Verification items for the finished model (mm, model axes). Face numbers are marked on the shaded views. A direction names the side the tool comes from. Coordinates: 2 decimals unless noted, no trailing zeros. Write each loop counter-clockwise with the first axis right and the second up, starting at its lowest first coordinate (ties: lowest second). Pieces come first, ordered by that corner, then holes. Notation, with made-up numbers: (47, -23.5) -> (100, -23.5) arc R11 cw to (100, -9.5) -> close; hole circle Ø3 at (-38, 61). An arc over 180 degrees is marked (long way). Answer in a Markdown table with one row per item.
```python
from build123d import *

# Parameters (mm, degrees)
BOSS_EXTRUDE1_DEPTH     = 82.55
SKETCH4_W               = 139.7
SKETCH4_H               = 139.7
SKETCH4_W_2             = 114.3
SKETCH4_H_2             = 114.3
BOSS_EXTRUDE2_DEPTH     = 152.4
SKETCH5_R               = 12.7
CUT_EXTRUDE1_DEPTH      = 1
CUT_EXTRUDE1_DEPTH_BACK = 166.1
SKETCH6_R               = 12.7
CUT_EXTRUDE2_DEPTH      = 13.7
CUT_EXTRUDE2_DEPTH_BACK = 153.4
CUT_EXTRUDE4_DEPTH      = 1
CUT_EXTRUDE4_DEPTH_BACK = 166.1
BODY_MOVE_COPY1_ANGLE   = 90
BODY_MOVE_COPY2_ANGLE   = 90


with BuildPart() as part:
    # Sketch2 → Boss-Extrude1 (new body, symmetric)
    with BuildSketch(Plane(origin=(0, 0, 0), x_dir=(1, 0, 0), z_dir=(0, 1, 0))):
        Polygon((-50.8, 38.1), (76.2, 38.1), (76.2, -101.6), (-50.8, -101.6), (-50.8, -114.3), (88.9, -114.3), (88.9, 50.8), (-50.8, 50.8), align=None)
    extrude(amount=BOSS_EXTRUDE1_DEPTH, both=True)

    # Sketch4 → Boss-Extrude2 (add)
    with BuildSketch(Plane(origin=(88.9, 0, 0), x_dir=(0, 0, -1), z_dir=(1, 0, 0))):
        with Locations((-31.75, 0)):
            Rectangle(SKETCH4_W, SKETCH4_H)
        with Locations((-31.75, 0)):
            Rectangle(SKETCH4_W_2, SKETCH4_H_2, mode=Mode.SUBTRACT)
    extrude(amount=BOSS_EXTRUDE2_DEPTH)

    # Sketch5 → Cut-Extrude1 (cut, two sides)
    with BuildSketch(Plane.XY.offset(114.3)) as cut_extrude1_sk:
        Circle(SKETCH5_R)
    extrude(amount=CUT_EXTRUDE1_DEPTH, mode=Mode.SUBTRACT)
    extrude(cut_extrude1_sk.sketch, amount=-CUT_EXTRUDE1_DEPTH_BACK, mode=Mode.SUBTRACT)

    # Sketch6 → Cut-Extrude2 (cut, two sides)
    with BuildSketch(Plane(origin=(0, 69.85, 0), x_dir=(1, 0, 0), z_dir=(0, 1, 0))) as cut_extrude2_sk:
        with Locations((215.9, -31.75)):
            Circle(SKETCH6_R)
    extrude(amount=CUT_EXTRUDE2_DEPTH, mode=Mode.SUBTRACT)
    extrude(cut_extrude2_sk.sketch, amount=-CUT_EXTRUDE2_DEPTH_BACK, mode=Mode.SUBTRACT)

    # Sketch7 → Cut-Extrude4 (cut, two sides)
    with BuildSketch(Plane.XY.offset(114.3)) as cut_extrude4_sk:
        with BuildLine():
            Line((-20.374273833, 82.55), (-68.429055494, 82.55))
            Line((-68.429055494, 82.55), (-68.429055494, -82.55))
            Line((-68.429055494, -82.55), (-20.374273833, -82.55))
            ThreePointArc((-20.374273833, -82.55), (-60.854450977, 0), (-20.374273833, 82.55))
        make_face()
    extrude(amount=CUT_EXTRUDE4_DEPTH, mode=Mode.SUBTRACT)
    extrude(cut_extrude4_sk.sketch, amount=-CUT_EXTRUDE4_DEPTH_BACK, mode=Mode.SUBTRACT)


with BuildPart() as part_1:
    # Body-Move/Copy1: moved
    add(part.part.rotate(Axis((0, 0, 31.75025), (1, 0, 0)), BODY_MOVE_COPY1_ANGLE))


with BuildPart() as part_2:
    # Body-Move/Copy2: moved
    add(part_1.part.rotate(Axis((0, 0, 31.75025), (-1, 0, 0)), BODY_MOVE_COPY2_ANGLE))


solid = part_2.part
```
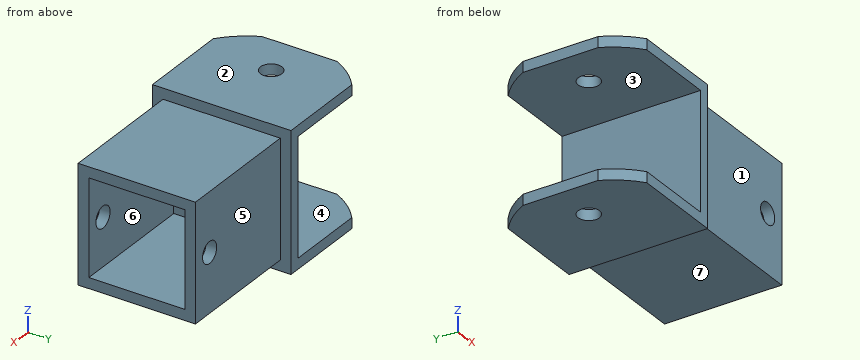
1. Depth check by flat-ended pin: P1, Ø6, axis at x = 176.5, z = 49.5, coming from the +Y side; P2, Ø5, axis at y = 28.5, z = 48.5, coming from the -X side; P3, Ø1.5, axis at x = 91, y = 51.5, coming from the -Z side. Enter the tip coordinate at first touch or a pass-through.
Geometry says:
| item | result |
|---|---|
| P1 | y = 69.85 |
| P2 | x = 76.2 |
| P3 | z = -38.1 |
2. Section check C-C, the plane z = 31.75. Record the boundary of the cut face in (x, y).
Geometry says:
| item | result |
|---|---|
| outline | (76.2, -82.55) -> (88.9, -82.55) -> (88.9, -69.85) -> (203.2, -69.85) -> (203.2, -57.15) -> (88.9, -57.15) -> (88.9, 57.15) -> (203.2, 57.15) -> (203.2, 69.85) -> (88.9, 69.85) -> (88.9, 82.55) -> (76.2, 82.55) -> close; (228.6, -69.85) -> (241.3, -69.85) -> (241.3, -57.15) -> (228.6, -57.15) -> close; (228.6, 57.15) -> (241.3, 57.15) -> (241.3, 69.85) -> (228.6, 69.85) -> close |
3. Section check D-D, the plane x = 0. Record the boundary of the cut face in (y, z).
Geometry says:
| item | result |
|---|---|
| outline | (-82.55, -50.8) -> (-12.7, -50.8) -> (-12.7, -38.1) -> (-82.55, -38.1) -> close; (-82.55, 101.6) -> (-12.7, 101.6) -> (-12.7, 114.3) -> (-82.55, 114.3) -> close; (12.7, -50.8) -> (82.55, -50.8) -> (82.55, -38.1) -> (12.7, -38.1) -> close; (12.7, 101.6) -> (82.55, 101.6) -> (82.55, 114.3) -> (12.7, 114.3) -> close |
4. Mould release check, pull along Z, two halves, no side actions. Record for the marked faces 1, 2 and 3: released by +Z, released by -Z, zero draft, split by the parting line, or undercut.
Geometry says:
| item | result |
|---|---|
| face 1 | zero draft |
| face 2 | released by +Z |
| face 3 | undercut |
5. Thickness scan on line 1 (Y direction, x = 0, z = -42); line 2 (Z direction, x = 215.9, y = 63); line 3 (Y direction, x = 113, z = 10.5). Record the ranges inside material, lowest first. Write a range as from..to.
Geometry says:
| item | result |
|---|---|
| line 1 | -82.55..-12.7, 12.7..82.55 |
| line 2 | -38.1..19.05, 44.45..101.6 |
| line 3 | -69.85..-57.15, 57.15..69.85 |
6. Section check B-B, the plane x = 215.9. Record the boundary of the cut face in (y, z).
Geometry says:
| item | result |
|---|---|
| outline | (-69.85, -38.1) -> (69.85, -38.1) -> (69.85, 19.05) -> (57.15, 19.05) -> (57.15, -25.4) -> (-57.15, -25.4) -> (-57.15, 19.05) -> (-69.85, 19.05) -> close; (-69.85, 44.45) -> (-57.15, 44.45) -> (-57.15, 88.9) -> (57.15, 88.9) -> (57.15, 44.45) -> (69.85, 44.45) -> (69.85, 101.6) -> (-69.85, 101.6) -> close |
7. Section check A-A, the plane y = 0. Record the boundary of the cut face in (x, z), plus the area to 3 significant figures.
Geometry says:
| item | result |
|---|---|
| outline | (-50.8, -50.8) -> (-12.7, -50.8) -> (-12.7, -38.1) -> (-50.8, -38.1) -> close; (-50.8, 101.6) -> (-12.7, 101.6) -> (-12.7, 114.3) -> (-50.8, 114.3) -> close; (12.7, -50.8) -> (88.9, -50.8) -> (88.9, -38.1) -> (241.3, -38.1) -> (241.3, -25.4) -> (88.9, -25.4) -> (88.9, 88.9) -> (241.3, 88.9) -> (241.3, 101.6) -> (88.9, 101.6) -> (88.9, 114.3) -> (12.7, 114.3) -> (12.7, 101.6) -> (76.2, 101.6) -> (76.2, -38.1) -> (12.7, -38.1) -> close |
| area | 8,550 mm^2 |
8. Tool access check on the marked faces 4, 5, 6 and 7. Record the directions out of +Z, -Z, +X, -X, +Y, -Y that give a thin tool (end or side, any length) a straight path to the whole face; none if there is none.
Geometry says:
| item | result |
|---|---|
| face 4 | -X, +Y, -Y |
| face 5 | +Z, -Z, +X, +Y |
| face 6 | +X |
| face 7 | -Z, +X, +Y, -Y |
